```python
from build123d import *

# Parameters (mm, degrees)
SKETCH2_R           = 1.6256
SKETCH2_R_2         = 1.143
BOSS_EXTRUDE1_DEPTH = 1.4859


with BuildPart() as part:
    # Sketch2 → Boss-Extrude1 (new body, symmetric)
    with BuildSketch(Plane.XY):
        with BuildLine():
            Line((1.669588526, -9.920736917), (14.750588526, -9.920736917))
            Line((14.750588526, -9.920736917), (15.004588526, -8.320536917))
            Line((15.004588526, -8.320536917), (11.730740811, -7.888736917))
            Line((11.730740811, -7.888736917), (11.730740811, -6.872736917))
            Line((11.730740811, -6.872736917), (6.533907217, -6.034536917))
            Line((6.533907217, -6.034536917), (6.533907217, 1.585463083))
            ThreePointArc((6.533907217, 1.585463083), (5.31342025, 4.700559773), (2.301635303, 6.157463083))
            Line((2.301635303, 6.157463083), (-5.77059015, 5.319263083))
            ThreePointArc((-5.77059015, 5.319263083), (-7.384864751, 4.650807821), (-8.371334953, 3.208728953))
            Line((-8.371334953, 3.208728953), (-11.346598434, -6.053267424))
            ThreePointArc((-11.346598434, -6.053267424), (-10.750121538, -8.941908183), (-7.96769015, -9.920736917))
            Line((-7.96769015, -9.920736917), (-3.57349015, -9.920736917))
            Line((-3.57349015, -9.920736917), (-3.850300754, -5.764344341))
            ThreePointArc((-3.850300754, -5.764344341), (-1.375609273, -3.046929144), (1.374211357, -5.485561912))
            Line((1.374211357, -5.485561912), (1.669588526, -9.920736917))
        make_face()
        with Locations((-8.493016303, -6.96993359)):
            Circle(SKETCH2_R, mode=Mode.SUBTRACT)
        with Locations((4.298707217, -5.475736917)):
            Circle(SKETCH2_R_2, mode=Mode.SUBTRACT)
    extrude(amount=BOSS_EXTRUDE1_DEPTH, both=True)


solid = part.part
```
Verification items for the finished model (mm, model axes). A direction names the side the tool comes from. Round coordinates to 2 decimals unless told otherwise and drop trailing zeros. Write each loop counter-clockwise with the first axis right and the second up, starting at its lowest first coordinate (ties: lowest second). Pieces come first, ordered by that corner, then holes. Notation, with made-up numbers: (-13, 28) - (17, 28) arc R20 cw to (17, 54) - close; hole circle Ø1 at (-12.75, -19.5). An arc over 180 degrees is marked (long way). Answer as a JSON object with one key per item and string values. Group by question number.
Q1. Tool access check on faces 4 (the flat face through (8, -9.921, 0)), 5 (the flat face through (1.52, -7.67, 0.02)), 6 (the flat face through (-3.71, -7.87, 0.02)), 7 (the flat face through (6.534, -2, 0)). Record the directions out of +Z, -Z, +X, -X, +Y, -Y that give a thin tool (end or side, any length) a straight path to the whole face; none if there is none.
Q2. Section check D-D, the plane y = 4. Enter the section's corners in (x, z).
Q3. Thickness scan on line 1 (X direction, y = -5.5, z = 0.35); line 2 (X direction, y = -4.5, z = 0.65); line 3 (Y direction, x = 4.5, z = 0.2). Record the ranges inside material, lowest first.
Q4. Section check C-C, the plane x = -1.5. Enter the section's corners in (y, z), plus the area to 3 significant figures.
Q5. Section check B-B, the plane z = -0.15. Enter the section's corners in (x, y).
Q6. Section check A-A, the plane y = -4. Enter the section's corners in (x, z), plus the area to 3 significant figures.
Q7. Go/stop test with a flat-tipped pin: pin 1 Ø1.5 at (y, z) = (-2.5, 0.5) entering from +X. Record where the tip stops, or that it passes through.
Q8. Mould release check, pull along Y, two halves, no side actions. Record for faces 1 (the flat face through (14.876, -9.132, 0.021)), 2 (the cylindrical face through (-9.69, -5.87, -0.02)), 3 (the flat face through (-1.678, 5.744, 0.021)): released by +Y, released by -Y, zero draft, split by the parting line, or undercut.
Found:
{
 "1": {"face 4": "+Z, -Z, +X, -Y", "face 5": "+Z, -Z, -Y", "face 6": "+Z, -Z", "face 7": "+Z, -Z, +X, +Y"},
 "2": {"outline": "(-7.98, -1.49) - (5.85, -1.49) - (5.85, 1.49) - (-7.98, 1.49) - close"},
 "3": {"line 1": "x = -11.17 to -9.19, -7.8 to -3.85, 1.38 to 3.16, 5.44 to 6.53", "line 2": "x = -10.85 to -3.58, 1.11 to 3.7, 4.89 to 6.53", "line 3": "y = -9.92 to -6.6, -4.35 to 5.4"},
 "4": {"outline": "(-3.06, -1.49) - (5.76, -1.49) - (5.76, 1.49) - (-3.06, 1.49) - close", "area": "26.2 mm^2"},
 "5": {"outline": "(-11.35, -6.05) arc R3 ccw to (-7.97, -9.92) - (-3.57, -9.92) - (-3.85, -5.76) arc R2.62 cw to (1.37, -5.49) - (1.67, -9.92) - (14.75, -9.92) - (15, -8.32) - (11.73, -7.89) - (11.73, -6.87) - (6.53, -6.03) - (6.53, 1.59) arc R4.59 ccw to (2.3, 6.16) - (-5.77, 5.32) arc R3.06 ccw to (-8.37, 3.21) - close; hole circle Ø3.25 at (-8.49, -6.97); hole circle Ø2.29 at (4.3, -5.48)"},
 "6": {"outline": "(-10.69, -1.49) - (-3.26, -1.49) - (-3.26, 1.49) - (-10.69, 1.49) - close; (0.79, -1.49) - (6.53, -1.49) - (6.53, 1.49) - (0.79, 1.49) - close", "area": "39.2 mm^2"},
 "7": {"pin 1": "stops at x = 6.53"},
 "8": {"face 1": "released by -Y", "face 2": "undercut", "face 3": "released by +Y"}
}
